from build123d import *

# Parameters (mm, degrees)
CROQUIS1_W                         = 8
CROQUIS1_H                         = 21
BRIDA_BASE1_DEPTH                  = 1
BRIDA_DE_ARISTA1_STRIP_W           = 5.4732
BRIDA_DE_ARISTA1_STRIP_H           = 1
BRIDA_DE_ARISTA1_STRIP_CUT_DEPTH   = 21
BRIDA_DE_ARISTA1_STRIP_2_W         = 5.4732
BRIDA_DE_ARISTA1_STRIP_2_H         = 1
BRIDA_DE_ARISTA1_STRIP_CUT_2_DEPTH = 21
BRIDA_DE_ARISTA1_DEPTH             = 21
BRIDA_DE_ARISTA1_BEND_DEPTH        = 21
CROQUIS34_W                        = 2
CROQUIS34_H                        = 7
CORTAR_EXTRUIR1_DEPTH              = 10
CORTAR_EXTRUIR2_REACH              = 16.714
CROQUIS35_R                        = 1
CORTAR_EXTRUIR3_DEPTH              = 10


# Sheet-metal steps are written as plain solids
with BuildPart() as part:
    # Croquis1 → Brida base1 (new body)
    with BuildSketch(Plane.XY):
        Rectangle(CROQUIS1_W, CROQUIS1_H)
    extrude(amount=-BRIDA_BASE1_DEPTH)

    # Brida de arista1 strip (across the edge) → Brida de arista1 strip cut (cut)
    with BuildSketch(Plane(origin=(-4, -10.5, -1), x_dir=(1, 0, 0), z_dir=(0, 1, 0))):
        with Locations((-1, -0.5)):
            Rectangle(BRIDA_DE_ARISTA1_STRIP_W, BRIDA_DE_ARISTA1_STRIP_H)
    extrude(amount=BRIDA_DE_ARISTA1_STRIP_CUT_DEPTH, mode=Mode.SUBTRACT)

    # Brida de arista1 strip 2 (across the edge) → Brida de arista1 strip cut 2 (cut)
    with BuildSketch(Plane(origin=(4, 10.5, -1), x_dir=(-1, 0, 0), z_dir=(0, -1, 0))):
        with Locations((-1, -0.5)):
            Rectangle(BRIDA_DE_ARISTA1_STRIP_2_W, BRIDA_DE_ARISTA1_STRIP_2_H)
    extrude(amount=BRIDA_DE_ARISTA1_STRIP_CUT_2_DEPTH, mode=Mode.SUBTRACT)

    # Brida de arista1 section (across the edge) → Brida de arista1 (add)
    with BuildSketch(Plane(origin=(-4, -10.5, -1), x_dir=(1, 0, 0), z_dir=(0, 1, 0))):
        with BuildLine():
            Line((0, 0.7366), (0, 5.5))
            Line((0, 5.5), (1, 5.5))
            Line((1, 5.5), (1, 0.7366))
            ThreePointArc((1, 0.7366), (1.215745145, 0.215745145), (1.7366, 0))
            Line((1.7366, 0), (1.7366, -1))
            ThreePointArc((1.7366, -1), (0.508638364, -0.491361636), (0, 0.7366))
        make_face()
    extrude(amount=BRIDA_DE_ARISTA1_DEPTH)

    # Brida de arista1 section 2 (across the edge) → Brida de arista1 bend (add)
    with BuildSketch(Plane(origin=(4, 10.5, -1), x_dir=(-1, 0, 0), z_dir=(0, -1, 0))):
        with BuildLine():
            Line((0, 0.7366), (0, 5.5))
            Line((0, 5.5), (1, 5.5))
            Line((1, 5.5), (1, 0.7366))
            ThreePointArc((1, 0.7366), (1.215745145, 0.215745145), (1.7366, 0))
            Line((1.7366, 0), (1.7366, -1))
            ThreePointArc((1.7366, -1), (0.508638364, -0.491361636), (0, 0.7366))
        make_face()
    extrude(amount=BRIDA_DE_ARISTA1_BEND_DEPTH)

    # Croquis34 → Cortar-Extruir1 (cut)
    with BuildSketch(Plane(origin=(4, 0, 0), x_dir=(0, 0, -1), z_dir=(1, 0, 0))):
        with Locations((1, 7)):
            Rectangle(CROQUIS34_W, CROQUIS34_H)
        with Locations((1, -7)):
            Rectangle(CROQUIS34_W, CROQUIS34_H)
    extrude(amount=-CORTAR_EXTRUIR1_DEPTH, mode=Mode.SUBTRACT)

    # Cortar-Extruir2: up to this face of the body (flat: up to its plane)
    cortar_extruir2_end = Plane(part.part.faces().sort_by_distance((-4, 0, -4.204419709))[0])
    # Croquis35 → Cortar-Extruir2 (cut, up to the picked face)
    with BuildSketch(Plane(origin=(4, 0, 0), x_dir=(0, 0, -1), z_dir=(1, 0, 0)), mode=Mode.PRIVATE) as cortar_extruir2_sk1:
        with Locations((4.25, 8.8)):
            Circle(CROQUIS35_R)
    cortar_extruir2_tool1 = split(extrude(cortar_extruir2_sk1.sketch, amount=-CORTAR_EXTRUIR2_REACH, mode=Mode.PRIVATE), bisect_by=cortar_extruir2_end, keep=Keep.BOTH, mode=Mode.PRIVATE)
    # Croquis35 → Cortar-Extruir2 (cut, up to the picked face)
    with BuildSketch(Plane(origin=(4, 0, 0), x_dir=(0, 0, -1), z_dir=(1, 0, 0)), mode=Mode.PRIVATE) as cortar_extruir2_sk2:
        with Locations(Location((4.25, -8.8, 0), (0, 0, 180))):
            Circle(CROQUIS35_R)
    cortar_extruir2_tool2 = split(extrude(cortar_extruir2_sk2.sketch, amount=-CORTAR_EXTRUIR2_REACH, mode=Mode.PRIVATE), bisect_by=cortar_extruir2_end, keep=Keep.BOTH, mode=Mode.PRIVATE)
    add(cortar_extruir2_tool1.solids().sort_by(Axis((4, 8.8, -4.25), (-1, 0, 0)))[0], mode=Mode.SUBTRACT)
    add(cortar_extruir2_tool2.solids().sort_by(Axis((4, -8.8, -4.25), (-1, 0, 0)))[0], mode=Mode.SUBTRACT)

    # Croquis36 → Cortar-Extruir3 (cut)
    with BuildSketch(Plane(origin=(4, 0, 0), x_dir=(0, 0, -1), z_dir=(1, 0, 0))):
        Polygon((0, 1.5), (3.377527081, 1.5), (6.5, -0.666434932), (6.5, 11.157411488), (0, 11.157411488), align=None)
    extrude(amount=-CORTAR_EXTRUIR3_DEPTH, mode=Mode.SUBTRACT)


solid = part.part
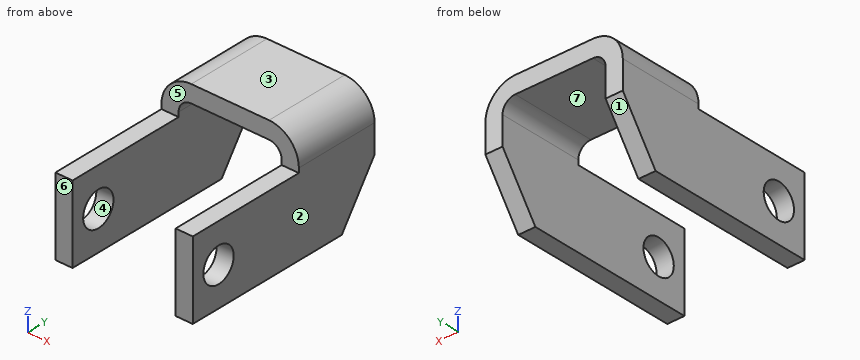
Here's how the part is built. I have some questions about the finished solid (model axes, mm). Face numbers are marked on the shaded views. A direction names the side the tool comes from. Give positions to 0.01 mm unless a question says otherwise; leave off trailing zeros. Order: outer loops, then holes, each group sorted by start corner. A loop starts at its lowest first (then second) coordinate and runs counter-clockwise, first axis right, second up. Notation, with made-up numbers: (26.25, 13.5) -> (75.25, 13.5) arc R28 ccw to (75.25, 35.5) -> close; hole circle Ø7 at (84, 36.5). An arc over 180 degrees is marked (long way). Use a Markdown table: item, result. Add a question column.
Item 1: Will these pins go through, and if not, where does the flat tip stop? pin 1 (1.5 mm diameter, centred on x = -1, z = -4, fed in from +Y); pin 2 (2 mm diameter, centred on x = 1.5, z = -1, fed in from -Y); pin 3 (3.5 mm diameter, centred on x = 0, y = -2, fed in from -Z); pin 4 (4 mm diameter, centred on x = 2.5, y = -7, fed in from +Z).
Item 2: I need wall thicknesses on line 1 (X direction, y = -5, z = -2.5); line 2 (Z direction, x = -3.55, y = -8.8); line 3 (Z direction, x = 0.5, y = -1.75). Which ranges of each line are inside material? Lowest first, please.
Item 3: If we mould it in two halves opening along Z, with no side actions, what happens to the marked faces 1, 2, 3 and 4? For each: pulls with the +Z half, pulls with the -Z half, needs draft (parallel to the pull), parting line crosses it, or undercut.
Item 4: Imagine slicing it at D-D on x = 3.75. Please give me the cut outline in (y, z).
Item 5: Imagine slicing it at A-A on y = -6.25. Please give me the cut outline in (x, z), plus the area to 3 significant figures.
Item 6: Imagine slicing it at B-B on z = -4.25. Please give me the cut outline in (x, y).
Item 7: Imagine slicing it at C-C on y = -8.8. Please give me the cut outline in (x, z), plus the area to 3 significant figures.
Item 8: For the marked faces 5, 6 and 7, which set-ups out of +Z, -Z, +X, -X, +Y, -Y let a thin tool reach every point of the face, with its end or its side?
Data:
| question | item | result |
|---|---|---|
| 1 | pin 1 | passes through |
| 1 | pin 2 | stops at y = -3.5 |
| 1 | pin 3 | stops at z = -1 |
| 1 | pin 4 | stops at z = -2 |
| 2 | line 1 | x = -4 to -3, 3 to 4 |
| 2 | line 2 | z = -6.5 to -5.25, -3.25 to -2 |
| 2 | line 3 | z = -1 to 0 |
| 3 | face 1 | pulls with the -Z half |
| 3 | face 2 | needs draft |
| 3 | face 3 | pulls with the +Z half |
| 3 | face 4 | undercut |
| 4 | outline | (-10.5, -6.5) -> (-0.67, -6.5) -> (1.5, -3.38) -> (1.5, -0.84) -> (-3.5, -0.84) -> (-3.5, -2) -> (-10.5, -2) -> close; hole circle Ø2 at (-8.8, -4.25) |
| 5 | outline | (-4, -6.5) -> (-3, -6.5) -> (-3, -2) -> (-4, -2) -> close; (3, -6.5) -> (4, -6.5) -> (4, -2) -> (3, -2) -> close |
| 5 | area | 9.00 mm² |
| 6 | outline | (-4, -10.5) -> (-3, -10.5) -> (-3, -9.8) -> (-4, -9.8) -> close; (-4, -7.8) -> (-3, -7.8) -> (-3, 0.89) -> (-4, 0.89) -> close; (3, -10.5) -> (4, -10.5) -> (4, -9.8) -> (3, -9.8) -> close; (3, -7.8) -> (4, -7.8) -> (4, 0.89) -> (3, 0.89) -> close |
| 7 | outline | (-4, -6.5) -> (-3, -6.5) -> (-3, -5.25) -> (-4, -5.25) -> close; (-4, -3.25) -> (-3, -3.25) -> (-3, -2) -> (-4, -2) -> close; (3, -6.5) -> (4, -6.5) -> (4, -5.25) -> (3, -5.25) -> close; (3, -3.25) -> (4, -3.25) -> (4, -2) -> (3, -2) -> close |
| 7 | area | 5.00 mm² |
| 8 | face 5 | +Z, +X, -X, -Y |
| 8 | face 6 | +Z, -Z, +X, -X, -Y |
| 8 | face 7 | -Z, +Y, -Y |
